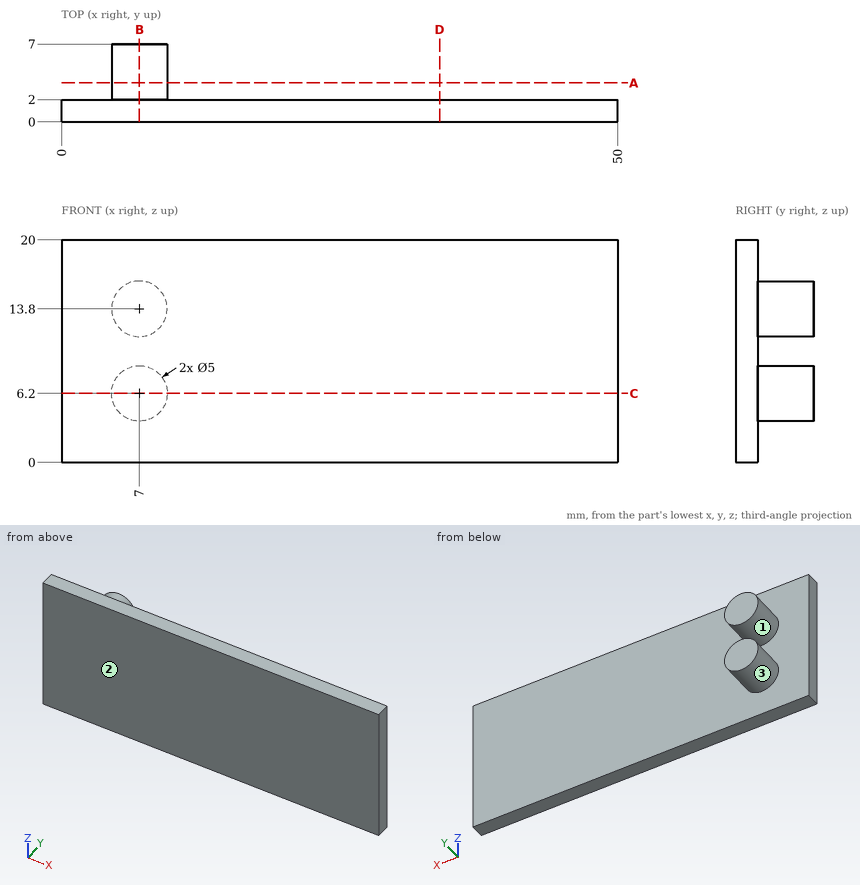
Could you check a few things on this drawing? It's one solid part, dimensions in mm from its lowest x, y, z. Give positions to 0.01 mm unless a question says otherwise; leave off trailing zeros. Loops run counter-clockwise (first coordinate to the right, second up) from the corner with the lowest first, then second, coordinate; pieces in that order, holes last. Notation, with made-up numbers: M 23,48 L 47,48 A22 ccw 47,58 Z; hole C 82.25,18.25 d1. An arc over 180 degrees is marked long. Answer as a JSON object with one key per item and string values.
Q1. For P1, Ø6, axis at x = 23, z = 6.5, coming from the +Y side; P2, Ø2, axis at y = 5, z = 12, coming from the -X side, each with a flat end and sliding along its axis, tell me the tip position at first contact or that it passes through.
Values found:
{"P1": "stops at y = 2", "P2": "stops at x = 4.63"}
Q2. Suppose I cut it at D-D, the plane x = 34. List the corners of the cut face in (y, z) for me.
Values found:
{"outline": "M 0,0 L 2,0 L 2,20 L 0,20 Z"}
Q3. Suppose I cut it at C-C, the plane z = 6.2. List the corners of the cut face in (x, y) for me.
Values found:
{"outline": "M 0,0 L 50,0 L 50,2 L 9.5,2 L 9.5,7 L 4.5,7 L 4.5,2 L 0,2 Z"}
Q4. Suppose I cut it at B-B, the plane x = 7. List the corners of the cut face in (y, z) for me.
Values found:
{"outline": "M 0,0 L 2,0 L 2,3.7 L 7,3.7 L 7,8.7 L 2,8.7 L 2,11.3 L 7,11.3 L 7,16.3 L 2,16.3 L 2,20 L 0,20 Z"}
Q5. Suppose I cut it at A-A, the plane y = 3.5. List the corners of the cut face in (x, z) for me, plus the area to 3 significant figures.
Values found:
{"outline": "C 7,6.2 d5; C 7,13.8 d5", "area": "39.3 mm²"}
Q6. If we mould it in two halves opening along Z, with no side actions, what happens to the marked faces 1, 2 and 3? For each: pulls with the +Z half, pulls with the -Z half, needs draft (parallel to the pull), parting line crosses it, or undercut.
Values found:
{"face 1": "undercut", "face 2": "needs draft", "face 3": "undercut"}
Q7. If I drill on probe 1 along Y at (x, z) = (22, 15.25); probe 2 along Z at (x, y) = (8.5, 2.25); probe 3 along X at (y, z) = (4, 14), over which ranges is the centre line in solid material (lowest first)? Write a range as [from, to].
Values found:
{"probe 1": "y = [0, 2]", "probe 2": "z = [4.2, 8.2], [11.8, 15.8]", "probe 3": "x = [4.51, 9.49]"}
